Work out the finished part from the listing and answer in its coordinate system (mm). A direction names the side the tool comes from. Give positions to 0.01 mm unless a question says otherwise; leave off trailing zeros. Loops run counter-clockwise (first coordinate to the right, second up) from the corner with the lowest first, then second, coordinate; pieces in that order, holes last.
from build123d import *

# Parameters (mm, degrees)
BOX004_W          = 8
BOX004_H          = 8
BOX004_DEPTH      = 9
CYLINDER_R        = 1
CYLINDER_DEPTH    = 10
CYLINDER001_R     = 1
CYLINDER001_DEPTH = 10
CYLINDER002_R     = 4.5
CYLINDER002_DEPTH = 12
CYLINDER003_R     = 4.5
CYLINDER003_DEPTH = 12
BOX002_W          = 5
BOX002_H          = 14
BOX002_DEPTH      = 11
BOX_W             = 15.2
BOX_H             = 68.2
BOX_DEPTH         = 18
BOX001_W          = 17
BOX001_H          = 70
BOX001_DEPTH      = 14
CHAMFER_SIZE      = 0.7
CHAMFER001_SIZE   = 0.7
CHAMFER002_SIZE   = 0.4
CHAMFER003_SIZE   = 0.4
CHAMFER004_SIZE   = 0.4


with BuildPart() as cubo003:
    # Box004 → Box004 (new body)
    with BuildSketch(Plane(origin=(-5, 8, -2), x_dir=(1, 0, 0), z_dir=(0, 0, 1))):
        with Locations((4, 4)):
            Rectangle(BOX004_W, BOX004_H)
    extrude(amount=BOX004_DEPTH)


with BuildPart() as led1:
    # Cylinder → Cylinder (new body)
    with BuildSketch(Plane(origin=(-5, 59, 7), x_dir=(0, 0, -1), z_dir=(1, 0, 0))):
        Circle(CYLINDER_R)
    extrude(amount=CYLINDER_DEPTH)


with BuildPart() as cilindro:
    # Cylinder001 → Cylinder001 (new body)
    with BuildSketch(Plane(origin=(-5, 53, 7), x_dir=(0, 0, -1), z_dir=(1, 0, 0))):
        Circle(CYLINDER001_R)
    extrude(amount=CYLINDER001_DEPTH)


with BuildPart() as cilindro001:
    # Cylinder002 → Cylinder002 (new body)
    with BuildSketch(Plane(origin=(-8, 8, 2.5), x_dir=(0, 0, -1), z_dir=(1, 0, 0))):
        Circle(CYLINDER002_R)
    extrude(amount=CYLINDER002_DEPTH)


with BuildPart() as fusion:
    # Cylinder003 → Cylinder003 (new body)
    with BuildSketch(Plane(origin=(-8, 17, 2.5), x_dir=(0, 0, -1), z_dir=(1, 0, 0))):
        Circle(CYLINDER003_R)
    extrude(amount=CYLINDER003_DEPTH)

    # Fusion: union Cilindro001
    add(cilindro001.part)


with BuildPart() as cubo001:
    # Box002 → Box002 (new body)
    with BuildSketch(Plane(origin=(1, 26, 2), x_dir=(1, 0, 0), z_dir=(0, 0, 1))):
        with Locations((2.5, 7)):
            Rectangle(BOX002_W, BOX002_H)
    extrude(amount=BOX002_DEPTH)


with BuildPart() as foroslot:
    # Box → Box (new body)
    with BuildSketch(Plane(origin=(-0.1, -0.1, -9), x_dir=(1, 0, 0), z_dir=(0, 0, 1))):
        with Locations((7.6, 34.1)):
            Rectangle(BOX_W, BOX_H)
    extrude(amount=BOX_DEPTH)


with BuildPart() as cut006:
    # Box001 → Box001 (new body)
    with BuildSketch(Plane(origin=(-1, -1, -4), x_dir=(1, 0, 0), z_dir=(0, 0, 1))):
        with Locations((8.5, 35)):
            Rectangle(BOX001_W, BOX001_H)
    extrude(amount=BOX001_DEPTH)

    # Cut: cut foroSlot
    add(foroslot.part, mode=Mode.SUBTRACT)

    # Cut001: cut Cubo001
    add(cubo001.part, mode=Mode.SUBTRACT)

    # Chamfer
    chamfer_edges = [cut006.edges().sort_by_distance(p)[0] for p in [
        (3.5, 26, 10),
        (6, 33, 10),
        (3.5, 40, 10),
        (1, 33, 10),
    ]]
    chamfer(chamfer_edges, length=CHAMFER_SIZE)

    # Chamfer001
    chamfer001_edges = [cut006.edges().sort_by_distance(p)[0] for p in [
        (-1, 34, 10),
        (7.5, -1, 10),
        (16, 34, 10),
        (7.5, 69, 10),
    ]]
    chamfer(chamfer001_edges, length=CHAMFER001_SIZE)

    # Cut002: cut Fusion
    add(fusion.part, mode=Mode.SUBTRACT)

    # Cut003: cut Cilindro
    add(cilindro.part, mode=Mode.SUBTRACT)

    # Cut004: cut Led1
    add(led1.part, mode=Mode.SUBTRACT)

    # Chamfer002
    chamfer002_edges = [cut006.edges().sort_by_distance(p)[0] for p in [
        (7.5, -1, -4),
        (7.5, 69, -4),
    ]]
    chamfer(chamfer002_edges, length=CHAMFER002_SIZE)

    # Chamfer003
    chamfer003_edges = [cut006.edges().sort_by_distance(p)[0] for p in [
        (-1, 34, -4),
        (16, 34, -4),
    ]]
    chamfer(chamfer003_edges, length=CHAMFER003_SIZE)

    # Chamfer004
    chamfer004_edges = [cut006.edges().sort_by_distance(p)[0] for p in [
        (-1, 69, 2.85),
        (-1, -1, 2.85),
        (16, -1, 2.85),
        (16, 69, 2.85),
    ]]
    chamfer(chamfer004_edges, length=CHAMFER004_SIZE)

    # Cut006: cut Cubo003
    add(cubo003.part, mode=Mode.SUBTRACT)


solid = cut006.part
Item 1: Find section A-A, the plane y = 17. Write down the section's boundary in (x, z), plus the area to 4 significant figures.
Item 2: Determine the mould class of faces 1 (the face through (7, 34, 10)), 2 (the face through (7, 69, 3)), 3 (the face through (-0.6, 21.5, 2.4)) for opening direction Z: released by +Z, released by -Z, zero draft, split by the parting line, or undercut.
Item 3: A flat-ended cylindrical pin translates along its axis: pin 1 Ø1 at (x, y) = (10.5, 19.5) entering from -Z. Find the tip coordinate at first contact, or state that the pin passes through.
Item 4: For faces 4 (the face through (7, 34, 9)), 5 (the face through (-0.6, 3.5, 2.6)), 6 (the face through (15.3, 34.2, -4)), determine the directions among +Z, -Z, +X, -X, +Y, -Y from which every point of the face is accessible in a straight line to the end or side of a thin tool.
Item 5: Find section B-B, the plane z = 2.5. Write down the section's boundary in (x, y), plus the area to 3 significant figures.
Item 6: Find section D-D, the plane x = 8.5. Write down the section's boundary in (y, z).
Item 7: Find section C-C, the plane y = 55.5. Write down the section's boundary in (x, z), plus the area to 4 significant figures.
Item 8: Consider line 1 (Y direction, x = 7, z = 1); line 2 (X direction, y = 35, z = 8); line 3 (Z direction, x = 1, y = 48). Determine where each line is inside the solid, lowest interval first.
Ans:
1. outline: (-1, -3.6) - (-0.6, -4) - (-0.1, -4) - (-0.1, -2) - (-1, -2) - close; (-1, 7) - (-0.1, 7) - (-0.1, 9) - (15.1, 9) - (15.1, -4) - (15.6, -4) - (16, -3.6) - (16, 9.3) - (15.3, 10) - (-0.3, 10) - (-1, 9.3) - close
1. area: 31.65 mm2
2. face 1: released by +Z
2. face 2: zero draft
2. face 3: undercut
3. pin 1: stops at z = 9
4. face 4: -Z
4. face 5: -X
4. face 6: -Z, +X, -X, +Y, -Y
5. outline: (-1, -0.6) - (-0.6, -1) - (15.6, -1) - (16, -0.6) - (16, 68.6) - (15.6, 69) - (-0.6, 69) - (-1, 68.6) - (-1, 21.5) - (-0.1, 21.5) - (-0.1, 68.1) - (15.1, 68.1) - (15.1, -0.1) - (-0.1, -0.1) - (-0.1, 3.5) - (-1, 3.5) - close
5. area: 137 mm2
6. outline: (-1, -3.6) - (-0.6, -4) - (-0.1, -4) - (-0.1, 9) - (68.1, 9) - (68.1, -4) - (68.6, -4) - (69, -3.6) - (69, 9.3) - (68.3, 10) - (-0.3, 10) - (-1, 9.3) - close
7. outline: (-1, -3.6) - (-0.6, -4) - (-0.1, -4) - (-0.1, 9) - (15.1, 9) - (15.1, -4) - (15.6, -4) - (16, -3.6) - (16, 9.3) - (15.3, 10) - (-0.3, 10) - (-1, 9.3) - close
7. area: 39.75 mm2
8. line 1: y = -1 to -0.1, 68.1 to 69
8. line 2: x = -1 to -0.1, 15.1 to 16
8. line 3: z = 9 to 10
